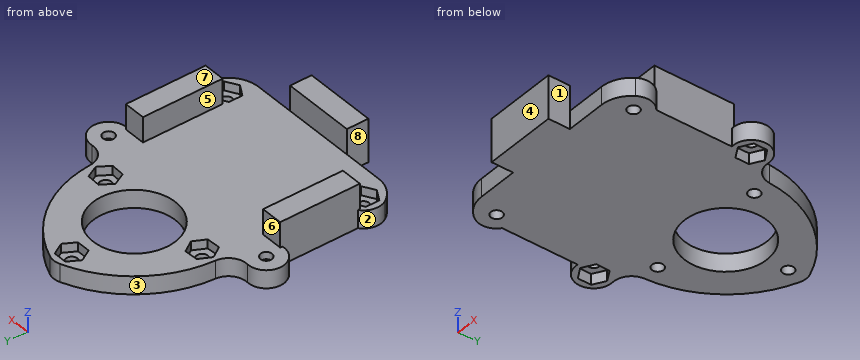
Autodesk Inventor part; units mm, degrees
ref_plane "YZ Plane" through (0, 0, 0) normal (1, 0, 0) x (0, 1, 0)
ref_plane "XZ Plane" through (0, 0, 0) normal (0, 1, 0) x (-1, 0, 0)
ref_plane "XY Plane" through (0, 0, 0) normal (0, 0, 1) x (1, 0, 0)
sketch "Sketch1" plane through (0, 0, 0) normal (0, 0, 1) x (1, 0, 0)
  circle A0 centre (0, 0) radius 11.5
  line L0 (21.15, -51.53) -> (-21.15, -51.53) construction
  line L1 (-21.15, -51.53) -> (-21.15, -9.23) construction
  line L2 (-21.15, -9.23) -> (21.15, -9.23) construction
  line L3 (21.15, -9.23) -> (21.15, -51.53) construction
  circle A1 centre (0, 17.5) radius 1.6
  circle A2 centre (17, -5.5) radius 1.6
  circle A3 centre (-17, -5.5) radius 1.6
  line L4 (13.2517, -5.3162) -> (15.2851, -2.162)
  line L5 (15.2851, -2.162) -> (19.0333, -2.3458)
  line L6 (19.0333, -2.3458) -> (20.7483, -5.6838)
  line L7 (20.7483, -5.6838) -> (18.7149, -8.838)
  line L8 (18.7149, -8.838) -> (14.9667, -8.6542)
  line L9 (14.9667, -8.6542) -> (13.2517, -5.3162)
  line L10 (-14.9667, -8.6542) -> (-18.7149, -8.838)
  line L11 (-18.7149, -8.838) -> (-20.7483, -5.6838)
  line L12 (-20.7483, -5.6838) -> (-19.0333, -2.3458)
  line L13 (-19.0333, -2.3458) -> (-15.2851, -2.162)
  line L14 (-15.2851, -2.162) -> (-13.2517, -5.3162)
  line L15 (-13.2517, -5.3162) -> (-14.9667, -8.6542)
  line L16 (-1.8764, 14.25) -> (-3.7528, 17.5)
  line L17 (-3.7528, 17.5) -> (-1.8764, 20.75)
  line L18 (-1.8764, 20.75) -> (1.8764, 20.75)
  line L19 (1.8764, 20.75) -> (3.7528, 17.5)
  line L20 (3.7528, 17.5) -> (1.8764, 14.25)
  line L21 (1.8764, 14.25) -> (-1.8764, 14.25)
  line L22 (0, 0) -> (0, 17.5) construction
  line L23 (14.9667, -8.6542) -> (14.9667, -9.23) construction
  line L24 (13.2517, -5.3162) -> (12.7488, -5.0358) construction
  line L25 (21.15, -41.53) -> (27.15, -41.53)
  line L26 (27.15, -41.53) -> (27.15, -19.23)
  line L27 (27.15, -19.23) -> (21.15, -19.23)
  line L28 (21.15, -19.23) -> (21.15, -41.53)
  line L29 (-21.15, -41.53) -> (-27.15, -41.53)
  line L30 (-27.15, -41.53) -> (-27.15, -19.23)
  line L31 (-27.15, -19.23) -> (-21.15, -19.23)
  line L32 (-21.15, -19.23) -> (-21.15, -41.53)
  circle A4 centre (27.75, -14.88) radius 1.6
  circle A5 centre (-27.75, -14.88) radius 1.6
  line L33 (24.5, -16.7564) -> (24.5, -13.0036)
  line L34 (24.5, -13.0036) -> (27.75, -11.1272)
  line L35 (27.75, -11.1272) -> (31, -13.0036)
  line L36 (31, -13.0036) -> (31, -16.7564)
  line L37 (31, -16.7564) -> (27.75, -18.6328)
  line L38 (27.75, -18.6328) -> (24.5, -16.7564)
  line L39 (-27.75, -18.6328) -> (-31, -16.7564)
  line L40 (-31, -16.7564) -> (-31, -13.0036)
  line L41 (-31, -13.0036) -> (-27.75, -11.1272)
  line L42 (-27.75, -11.1272) -> (-24.5, -13.0036)
  line L43 (-24.5, -13.0036) -> (-24.5, -16.7564)
  line L44 (-24.5, -16.7564) -> (-27.75, -18.6328)
  circle A6 centre (-24.1, -44.9364) radius 1.6
  circle A7 centre (24.1, -44.9364) radius 1.6
  line L45 (-24.1, -48.6891) -> (-27.35, -46.8128)
  line L46 (-27.35, -46.8128) -> (-27.35, -43.06)
  line L47 (-27.35, -43.06) -> (-24.1, -41.1836)
  line L48 (-24.1, -41.1836) -> (-20.85, -43.06)
  line L49 (-20.85, -43.06) -> (-20.85, -46.8128)
  line L50 (-20.85, -46.8128) -> (-24.1, -48.6891)
  line L51 (24.1, -48.6891) -> (20.85, -46.8128)
  line L52 (20.85, -46.8128) -> (20.85, -43.06)
  line L53 (20.85, -43.06) -> (24.1, -41.1836)
  line L54 (24.1, -41.1836) -> (27.35, -43.06)
  line L55 (27.35, -43.06) -> (27.35, -46.8128)
  line L56 (27.35, -46.8128) -> (24.1, -48.6891)
  arc A8 (-27.3663, -9.8947) -> (-27.15, -19.8439) centre (-27.75, -14.88) ccw
  arc A9 (27.15, -19.8439) -> (27.3663, -9.8947) centre (27.75, -14.88) ccw
  arc A10 (-27.15, -40.9744) -> (-28.2818, -47.6773) centre (-24.1, -44.9364) ccw
  arc A11 (28.2818, -47.6773) -> (27.15, -40.9744) centre (24.1, -44.9364) ccw
  line L57 (21.15, -48.9734) -> (21.15, -51.53)
  line L58 (21.15, -51.53) -> (-21.15, -51.53)
  line L59 (-21.15, -51.53) -> (-21.15, -48.9734)
  arc A12 (1.7467, 22.185) -> (-1.7467, 22.185) centre (0, 17.5) ccw
  arc A13 (-27.3663, -9.8947) -> (-21.9913, -5.2047) centre (-26.9825, -4.9095) ccw
  arc A14 (21.9913, -5.2047) -> (27.3663, -9.8947) centre (26.9825, -4.9095) ccw
  arc A15 (21.15, -51.53) -> (28.2818, -47.6773) centre (21.15, -43.0028) ccw
  arc A16 (-28.2818, -47.6773) -> (-21.15, -51.53) centre (-21.15, -43.0028) ccw
  arc A17 (-1.7467, 22.185) -> (-21.9913, -5.2047) centre (9.1518, -7.047) ccw
  arc A18 (21.9913, -5.2047) -> (1.7467, 22.185) centre (-9.1518, -7.047) ccw
  dimension "d1" = 23
  dimension "d19" = 9.23
  dimension "d20" = 42.3
  dimension "d21" = 21.15
  dimension "d22" = 42.3
  dimension "d23" = 3.2
  dimension "d24" = 3.2
  dimension "d25" = 3.2
  dimension "d26" = 5.5
  dimension "d27" = 17
  dimension "d28" = 5.5
  dimension "d29" = 17
  dimension "d30" = 6.5
  dimension "d31" = 17.5
  dimension "d32" = 6.5
  dimension "d33" = 6.5
  dimension "d35" = 0.5758
  dimension "d36" = 0.5758
  dimension "d37" = 6
  dimension "d38" = 10
  dimension "d39" = 10
  dimension "d40" = 6
  dimension "d41" = 3.2
  dimension "d42" = 3.2
  dimension "d43" = 5.65
  dimension "d44" = 6.6
  dimension "d45" = 6.6
  dimension "d46" = 5.65
  dimension "d47" = 6.5
  dimension "d48" = 6.5
  dimension "d49" = 3.2
  dimension "d50" = 3.2
  dimension "d52" = 2.95
  dimension "d53" = 2.95
  dimension "d56" = 10
  dimension "d57" = 10
  dimension "d58" = 10
  dimension "d59" = 10
  dimension "d61" = 10
  dimension "d63" = 10
  dimension "d64" = 10
  dimension "d90" = 3.4064
  dimension "d91" = 3.4064
  dimension "d92" = 6.5
  dimension "d93" = 6.5
extrude "Extrusion5" add sketch "Sketch1" along normal blind 5 contours L25 L53 L52 L51 L56 L55 L54 L26 A11 A15 L58 A16 A10 L30 L29 L47 L46 L45 L50 L49 L48 L32 L31 A8 A13 A17 A12 A18 A14 A9 L27 L28 | L33 L34 L35 L36 L37 L38 | L39 L40 L41 L42 L43 L44
extrude "Extrusion6" add sketch "Sketch1" along normal blind 12 contours L28 L27 L26 L25 L54 L53 | L53 L54 L25 | L30 L31 L32 L29 L48 L47 | L47 L48 L29
extrude "Extrusion7" add sketch "Sketch1" along normal blind 2.5 contours L4 L5 L6 L7 L8 L9 | L10 L11 L12 L13 L14 L15 | L16 L17 L18 L19 L20 L21 | L53 L54 L25 | L25 L54 L55 L56 L51 L52 L53 | L47 L48 L29 | L29 L48 L49 L50 L45 L46 L47
extrude "Extrusion8" cut sketch "Sketch1" along normal blind 3 contours L33 L34 L35 L36 L37 L38 | L39 L40 L41 L42 L43 L44
sketch "Sketch2" plane through (0, 0, 5) normal (0, 0, 1) x (1, 0, 0)
  circle A0 centre (0, 17.5) radius 1.6
  circle A1 centre (-17, -5.5) radius 1.6
  circle A2 centre (-17, -5.5) radius 1.6
  circle A3 centre (-24.1, -44.9364) radius 1.6
  circle A4 centre (24.1, -44.9364) radius 1.6
  circle A5 centre (24.1, -44.9364) radius 1.6
  circle A6 centre (17, -5.5) radius 1.6
  circle A7 centre (17, -5.5) radius 1.6
  circle A8 centre (0, 0) radius 11.5
  circle A9 centre (0, 0) radius 11.5
  dimension "d77" = 23
  dimension "d78" = 17.5
  dimension "d79" = 34
  dimension "d80" = 5.5
  dimension "d81" = 48.2
  dimension "d82" = 44.9364
sketch "Sketch3" plane through (0, 0, 5) normal (0, 0, 1) x (1, 0, 0)
  circle A0 centre (-27.75, -14.88) radius 1.6
  circle A1 centre (27.75, -14.88) radius 1.6
  circle A2 centre (0, 0) radius 11.5
  line L0 (-3.7528, 17.5) -> (-1.8764, 20.75)
  line L1 (-1.8764, 20.75) -> (1.8764, 20.75)
  line L2 (1.8764, 20.75) -> (3.7528, 17.5)
  line L3 (3.7528, 17.5) -> (1.8764, 14.25)
  line L4 (1.8764, 14.25) -> (-1.8764, 14.25)
  line L5 (-1.8764, 14.25) -> (-3.7528, 17.5)
  line L6 (-18.7149, -8.838) -> (-20.7483, -5.6838)
  line L7 (-20.7483, -5.6838) -> (-19.0333, -2.3458)
  line L8 (-19.0333, -2.3458) -> (-15.2851, -2.162)
  line L9 (-15.2851, -2.162) -> (-13.2517, -5.3162)
  line L10 (-13.2517, -5.3162) -> (-14.9667, -8.6542)
  line L11 (-14.9667, -8.6542) -> (-18.7149, -8.838)
  line L12 (15.2851, -2.162) -> (19.0333, -2.3458)
  line L13 (19.0333, -2.3458) -> (20.7483, -5.6838)
  line L14 (20.7483, -5.6838) -> (18.7149, -8.838)
  line L15 (18.7149, -8.838) -> (14.9667, -8.6542)
  line L16 (14.9667, -8.6542) -> (13.2517, -5.3162)
  line L17 (13.2517, -5.3162) -> (15.2851, -2.162)
  arc A3 (21.15, -51.53) -> (28.2818, -47.6773) centre (21.15, -43.0028) ccw
  arc A4 (28.2818, -47.6773) -> (27.15, -40.9744) centre (24.1, -44.9364) ccw
  line L18 (27.15, -40.9744) -> (27.15, -41.53)
  line L19 (27.15, -41.53) -> (24.7, -41.53)
  line L20 (24.7, -41.53) -> (27.35, -43.06)
  line L21 (27.35, -43.06) -> (27.35, -46.8128)
  line L22 (27.35, -46.8128) -> (24.1, -48.6891)
  line L23 (24.1, -48.6891) -> (20.85, -46.8128)
  line L24 (20.85, -46.8128) -> (20.85, -43.06)
  line L25 (20.85, -43.06) -> (23.5, -41.53)
  line L26 (21.15, -41.53) -> (21.15, -19.23)
  line L27 (21.15, -19.23) -> (27.15, -19.23)
  line L28 (27.15, -19.23) -> (27.15, -19.8439)
  arc A5 (27.15, -19.8439) -> (27.3663, -9.8947) centre (27.75, -14.88) ccw
  arc A6 (21.9913, -5.2047) -> (27.3663, -9.8947) centre (26.9825, -4.9095) ccw
  arc A7 (21.9913, -5.2047) -> (1.7467, 22.185) centre (-9.1518, -7.047) ccw
  arc A8 (1.7467, 22.185) -> (-1.7467, 22.185) centre (0, 17.5) ccw
  arc A9 (-1.7467, 22.185) -> (-21.9913, -5.2047) centre (9.1518, -7.047) ccw
  arc A10 (-27.3663, -9.8947) -> (-21.9913, -5.2047) centre (-26.9825, -4.9095) ccw
  arc A11 (-27.3663, -9.8947) -> (-27.15, -19.8439) centre (-27.75, -14.88) ccw
  line L29 (-27.15, -19.8439) -> (-27.15, -19.23)
  line L30 (-27.15, -19.23) -> (-21.15, -19.23)
  line L31 (-21.15, -19.23) -> (-21.15, -41.53)
  line L32 (-24.7, -41.53) -> (-27.15, -41.53)
  line L33 (-23.5, -41.53) -> (-20.85, -43.06)
  line L34 (-20.85, -43.06) -> (-20.85, -46.8128)
  line L35 (-20.85, -46.8128) -> (-24.1, -48.6891)
  line L36 (-24.1, -48.6891) -> (-27.35, -46.8128)
  line L37 (-27.35, -46.8128) -> (-27.35, -43.06)
  line L38 (-27.35, -43.06) -> (-24.7, -41.53)
  line L39 (-27.15, -41.53) -> (-27.15, -40.9744)
  arc A12 (-27.15, -40.9744) -> (-28.2818, -47.6773) centre (-24.1, -44.9364) ccw
  arc A13 (-28.2818, -47.6773) -> (-21.15, -51.53) centre (-21.15, -43.0028) ccw
  line L40 (-21.15, -51.53) -> (21.15, -51.53)
  line L41 (-21.15, -51.53) -> (21.15, -51.53)
  line L42 (-10, -51.53) -> (10, -51.53)
  line L43 (10, -51.53) -> (10, -57.53)
  line L44 (10, -57.53) -> (-10, -57.53)
  line L45 (-10, -57.53) -> (-10, -51.53)
  line L46 (23.5, -41.53) -> (21.15, -41.53)
  line L47 (-21.15, -41.53) -> (-23.5, -41.53)
  dimension "d83" = 6
  dimension "d84" = 20
  dimension "d85" = 10
extrude "Extrusion9" add sketch "Sketch3" against normal blind 5 and the other way blind 7 contours L43 L44 L45 L40
equation "\"d22\" = d20"
properties part number "BallBearingHolderBottom"
Read the model definition and answer for the solid it produces. Units are mm, in the model's axes. Face numbers are marked on the shaded views. A direction names the side the tool comes from. Coordinates: 2 decimals unless noted, no trailing zeros. Order: outer loops, then holes, each group sorted by start corner. A loop starts at its lowest first (then second) coordinate and runs counter-clockwise, first axis right, second up. Notation, with made-up numbers: M 55.25,79 L 104.25,79 A16 ccw 104.25,100 Z; hole C 46,50 d3. An arc over 180 degrees is marked long. Put each result on its own line as item: value. Start each with the question number.
Item 1: The mould has two halves that part along Y. Classify the marked faces 1, 2 and 3: +Y half, -Y half, draft (parallel to the pull), parting line (faces both ways), or undercut.
Item 2: Section C-C, the plane y = -14.88 is taken. Determine the outline of the cut face in (x, z).
Item 3: Consider probe 1 along Y at (x, z) = (2, 3); probe 2 along X at (y, z) = (-17.5, 1); probe 3 along Y at (x, z) = (27.75, 4). Determine where each line is inside the solid, lowest interval first. Write a range as [from, to].
Item 4: For the marked faces 4, 5, 6, 7 and 8, determine the directions among +Z, -Z, +X, -X, +Y, -Y from which every point of the face is accessible in a straight line to the end or side of a thin tool.
Item 5: Section D-D, the plane y = -39 is taken. Determine the outline of the cut face in (x, z), plus the area to 4 significant figures.
Item 6: Section A-A, the plane z = 9.5 is taken. Determine the outline of the cut face in (x, y).
Item 7: Given pin 1 Ø1.5 at (y, z) = (-14, 2) entering from +X; pin 2 Ø2 at (x, y) = (21.5, -8.5) entering from +Z; pin 3 Ø1.8 at (x, z) = (-22.5, 9.5) entering from +Y, each flat-ended and moving along its own axis, determine where each tip first touches the part or whether it passes through.
Item 8: Section B-B, the plane x = 0 is taken. Determine the outline of the cut face in (y, z), plus the area to 3 significant figures.
Computed:
1. face 1: draft
1. face 2: undercut
1. face 3: +Y half
2. outline: M -32.75,0 L -31,0 L -31,3 L -29.35,3 L -29.35,5 L -32.75,5 Z; M -26.15,3 L -24.5,3 L -24.5,0 L 24.5,0 L 24.5,3 L 26.15,3 L 26.15,5 L -26.15,5 Z; M 29.35,3 L 31,3 L 31,0 L 32.75,0 L 32.75,5 L 29.35,5 Z
3. probe 1: y = [-57.53, -11.32], [11.32, 14.46], [20.54, 22.09]
3. probe 2: x = [-32.01, -29.71], [-25.79, 25.79], [29.71, 32.01]
3. probe 3: y = [-48.4, -41.52], [-19.88, -16.48], [-13.28, -9.88]
4. face 4: +Z, -Z, +X, -X, -Y
4. face 5: +Z, +Y, -Y
4. face 6: +Z, +X, -X, +Y
4. face 7: +Z, +X, -X, +Y, -Y
4. face 8: +Z, -Z, -X, -Y
5. outline: M -27.15,0 L 27.15,0 L 27.15,12 L 21.15,12 L 21.15,5 L -21.15,5 L -21.15,12 L -27.15,12 Z
5. area: 355.5 mm2
6. outline: M -27.15,-41.53 L -21.15,-41.53 L -21.15,-19.23 L -27.15,-19.23 Z; M -10,-57.53 L 10,-57.53 L 10,-51.53 L -10,-51.53 Z; M 21.15,-41.53 L 27.15,-41.53 L 27.15,-19.23 L 21.15,-19.23 Z
7. pin 1: stops at x = 32.75
7. pin 2: stops at z = 5
7. pin 3: stops at y = -19.23
8. outline: M -57.53,0 L -11.5,0 L -11.5,5 L -51.53,5 L -51.53,12 L -57.53,12 Z; M 11.5,0 L 15.9,0 L 15.9,2.5 L 14.25,2.5 L 14.25,5 L 11.5,5 Z; M 19.1,0 L 22.5,0 L 22.5,5 L 20.75,5 L 20.75,2.5 L 19.1,2.5 Z
8. area: 303 mm2
